Geometry: final body of the model. Coordinates: model frame, mm. Face numbers are marked on the shaded views. A direction names the side the tool comes from. Round coordinates to 2 decimals unless told otherwise and drop trailing zeros. Loops run counter-clockwise (first coordinate to the right, second up) from the corner with the lowest first, then second, coordinate; pieces in that order, holes last. Notation, with made-up numbers: (58, 70.5) - (79, 70.5) arc R21 ccw to (79, 95.5) - close; hole circle Ø9 at (73.5, 69.5). An arc over 180 degrees is marked (long way). Return JSON: item names as keys, results as strings. Group by question number.
1. Set-up query: the marked faces 4, 5 and 6. Return all of +Z, -Z, +X, -X, +Y, -Y with unobstructed straight access to the full face (end or side cutting, diameter ignored); none if empty.
2. First-contact query: pin 1 Ø2 at (x, z) = (-5.5, -18.5) entering from -Y; pin 2 Ø3 at (x, y) = (-0.5, -3) entering from -Z; pin 3 Ø1.5 at (x, y) = (5.5, -2.5) entering from +Z. Flat tips, straight axial feed; report the tip coordinate or a pass-through.
3. Material intervals for probe 1 along X at (y, z) = (3, -33); probe 2 along Y at (x, z) = (-5.5, -30.5); probe 3 along Y at (x, z) = (2.5, -10), sorted ascending.
4. Section B-B on x = 1. Return loops of the section in (y, z), and give its area (3 significant figures).
5. Section A-A on z = -33. Return loops of the section in (x, y).
6. Draft query along X for the marked faces 1, 2 and 3. Return one class per face: +X half, -X half, draft (parallel to the pull), parting line (faces both ways), or undercut.
7. Section C-C on x = -5.75. Return loops of the section in (y, z).
8. Section D-D on z = -7. Return loops of the section in (x, y).
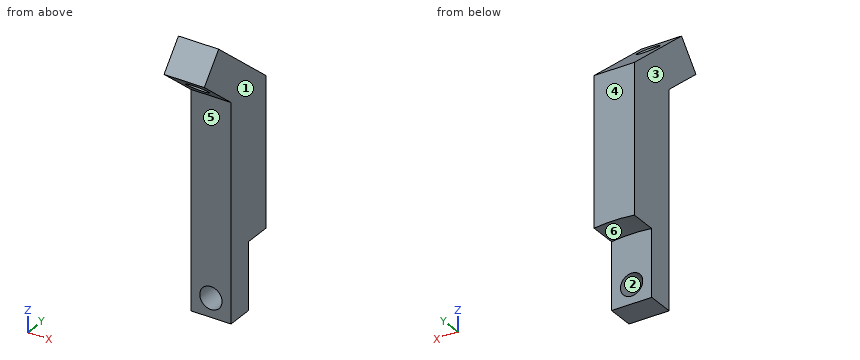
from build123d import *

# Parameters (mm, degrees)
SKETCH1_W           = 15
SKETCH1_H           = 80
SKETCH1_R           = 4.15
BOSS_EXTRUDE1_DEPTH = 10
BOSS_EXTRUDE2_DEPTH = 10
BOSS_EXTRUDE4_DEPTH = 15
SKETCH11_R          = 4
CUT_EXTRUDE5_DEPTH  = 31.247894791


with BuildPart() as part:
    # Sketch1 → Boss-Extrude1 (new body)
    with BuildSketch(Plane(origin=(0, 0, 0), x_dir=(1, 0, 0), z_dir=(0, 1, 0))):
        Rectangle(SKETCH1_W, SKETCH1_H)
        with Locations(Location((0, 33, 0), (0, 0, 270))):  # turned: the seam where the file's is
            Circle(SKETCH1_R, mode=Mode.SUBTRACT)
    extrude(amount=BOSS_EXTRUDE1_DEPTH)

    # Sketch2 → Boss-Extrude2 (add)
    with BuildSketch(Plane(origin=(0, 10, 0), x_dir=(1, 0, 0), z_dir=(0, 1, 0))):
        with BuildLine():
            Line((7.5, 15.134142149), (7.5, -40))
            Line((7.5, -40), (-7.5, -40))
            Line((-7.5, -40), (-7.5, 15.134142149))
            ThreePointArc((-7.5, 15.134142149), (0, 14.7), (7.5, 15.134142149))
        make_face()
    extrude(amount=BOSS_EXTRUDE2_DEPTH)

    # Sketch10 → Boss-Extrude4 (add)
    with BuildSketch(Plane(origin=(7.5, 0, 0), x_dir=(0, 0, -1), z_dir=(1, 0, 0))):
        Polygon((-40, 0), (-52.855752194, -15.320888862), (-62.703829724, -7.057370639), (-40, 20), align=None)
    extrude(amount=-BOSS_EXTRUDE4_DEPTH)

    # Sketch11 → Cut-Extrude5 (cut, through all)
    with BuildSketch(Plane(origin=(0, 19.69615506, 23.472963553), x_dir=(-1, 0, 0), z_dir=(0, -0.64278761, -0.766044443))):
        with Locations(Location((0, -35.711504387, 0), (0, 0, 90))):  # turned: the seam where the file's is
            Circle(SKETCH11_R)
    extrude(amount=-CUT_EXTRUDE5_DEPTH, mode=Mode.SUBTRACT)


solid = part.part
Taken from the geometry:
{
 "1": {"face 4": "+Z, -Z, +X, -X, +Y", "face 5": "-Z, +X, -X, -Y", "face 6": "-Z, +Y"},
 "2": {"pin 1": "y = 0", "pin 2": "z = 41.26", "pin 3": "z = 59.51"},
 "3": {"probe 1": "-7.5 to -4.15, 4.15 to 7.5", "probe 2": "0 to 10", "probe 3": "0 to 20"},
 "4": {"outline": "(-15.32, 52.86) - (-10.63, 48.92) - (-2.36, 58.77) - (-7.06, 62.7) - close; (-4.69, 43.94) - (0, 40) - (0, -28.97) - (10, -28.97) - (10, -14.71) - (20, -14.71) - (20, 40) - (3.57, 53.79) - close; (0, -40) - (10, -40) - (10, -37.03) - (0, -37.03) - close", "area": "1,520 mm2"},
 "5": {"outline": "(-7.5, 0) - (-4.15, 0) - (-4.15, 10) - (-7.5, 10) - close; (4.15, 0) - (7.5, 0) - (7.5, 10) - (4.15, 10) - close"},
 "6": {"face 1": "+X half", "face 2": "undercut", "face 3": "-X half"},
 "7": {"outline": "(-15.32, 52.86) - (0, 40) - (0, -40) - (10, -40) - (10, -14.95) - (20, -14.95) - (20, 40) - (-7.06, 62.7) - close"},
 "8": {"outline": "(-7.5, 0) - (7.5, 0) - (7.5, 20) - (-7.5, 20) - close"}
}
